Design review of the part built by this model. Coordinates are the model's own, in mm. Face numbers are marked on the shaded views. Give positions to 0.01 mm unless a question says otherwise; leave off trailing zeros. Use a Markdown table: item, result. Add a question column.
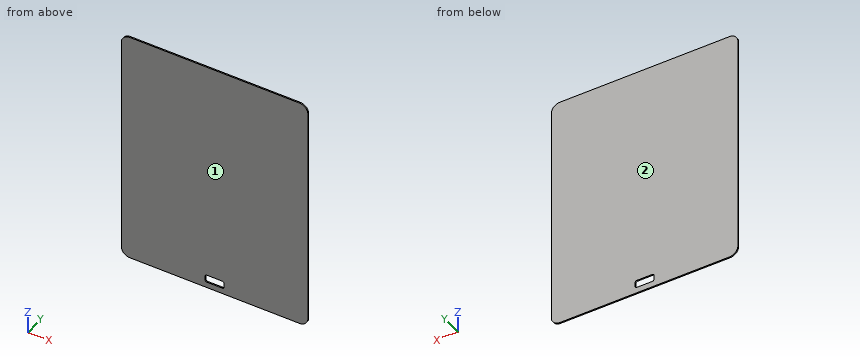
```python
from build123d import *

# Parameters (mm, degrees)
SKETCH1_W           = 217
SKETCH1_H           = 276.5
BOSS_EXTRUDE1_DEPTH = 1.5
FILLET1_R           = 10
SKETCH4_W           = 22
SKETCH4_H           = 8.75
CUT_EXTRUDE2_DEPTH  = 184.114035508
FILLET2_R           = 2


with BuildPart() as part:
    # Sketch1 → Boss-Extrude1 (new body)
    with BuildSketch(Plane(origin=(0, 0, 0), x_dir=(1, 0, 0), z_dir=(0, 1, 0))):
        with Locations((0, 9.25)):
            Rectangle(SKETCH1_W, SKETCH1_H)
    extrude(amount=BOSS_EXTRUDE1_DEPTH)

    # Fillet1
    fillet1_edges = [part.edges().sort_by_distance(p)[0] for p in [
        (-108.5, 0.75, -147.5),
        (108.5, 0.75, -147.5),
        (108.5, 0.75, 129),
        (-108.5, 0.75, 129),
    ]]
    fillet(fillet1_edges, radius=FILLET1_R)

    # Sketch4 → Cut-Extrude2 (cut, through all)
    with BuildSketch(Plane(origin=(0, 1.5, 0), x_dir=(1, 0, 0), z_dir=(0, 1, 0))):
        with Locations((0, 136.355)):
            Rectangle(SKETCH4_W, SKETCH4_H)
    extrude(amount=-CUT_EXTRUDE2_DEPTH, mode=Mode.SUBTRACT)

    # Fillet2
    fillet2_edges = [part.edges().sort_by_distance(p)[0] for p in [
        (-11, 0.75, -131.98),
        (-11, 0.75, -140.73),
        (11, 0.75, -140.73),
        (11, 0.75, -131.98),
    ]]
    fillet(fillet2_edges, radius=FILLET2_R)


solid = part.part
```
(1) Mouldability with a two-part tool opening along Y and no side actions: class the marked faces 1 and 2 as +Y half, -Y half, draft (parallel to the pull), parting line (faces both ways), or undercut.
(2) Insertion check: pin 1 (4 mm diameter, centred on x = 70, z = -96, fed in from -Y). The pin has a flat end and moves straight along its axis. Give the tip position at first contact, or say it passes through.
(3) For line 1 along Z through (x, y) = (-2.5, 1); line 2 along X through (y, z) = (0.65, -134), list the stretches that pass through material, from the lowest coordinate up.
Answers follow:
| question | item | result |
|---|---|---|
| 1 | face 1 | -Y half |
| 1 | face 2 | +Y half |
| 2 | pin 1 | y = 0 |
| 3 | line 1 | -147.5 to -140.73, -131.98 to 129 |
| 3 | line 2 | -108.5 to -11, 11 to 108.5 |
